from build123d import *

# Parameters (mm, degrees)
F0_R     = 5.5
F0_R_2   = 42
F1_DEPTH = 12


with BuildPart() as f1:
    # F0 (on Front) → F1 (new body)
    with BuildSketch(Plane.XZ):
        with BuildLine():
            ThreePointArc((-52.973189, -28.214553), (-49.277102, -27.650029), (-46.222895, -29.806777))
            ThreePointArc((-46.222895, -29.806777), (-32.248964, -44.553388), (-13.874959, -53.2211))
            ThreePointArc((-13.874959, -53.2211), (-10.872022, -55.44868), (-10.253636, -59.136137))
            ThreePointArc((-10.253636, -59.136137), (0, -71.897322), (10.253636, -59.136137))
            ThreePointArc((10.253636, -59.136137), (10.872022, -55.44868), (13.874959, -53.2211))
            ThreePointArc((13.874959, -53.2211), (32.248964, -44.553388), (46.222895, -29.806777))
            ThreePointArc((46.222895, -29.806777), (49.277102, -27.650029), (52.973189, -28.214553))
            ThreePointArc((52.973189, -28.214553), (68.298918, -22.460693), (59.379651, -8.733655))
            ThreePointArc((59.379651, -8.733655), (56.069932, -6.994258), (54.891958, -3.44572))
            ThreePointArc((54.891958, -3.44572), (47.477641, 27.764611), (23.912186, 49.529864))
            ThreePointArc((23.912186, 49.529864), (21.397105, 52.29647), (21.504018, 56.033891))
            ThreePointArc((21.504018, 56.033891), (13.913807, 70.538152), (1.384423, 60.002526))
            ThreePointArc((1.384423, 60.002526), (0.064118, 56.504449), (-3.313139, 54.900119))
            ThreePointArc((-3.313139, 54.900119), (-41.207009, 36.42777), (-54.891958, -3.44572))
            ThreePointArc((-54.891958, -3.44572), (-56.069932, -6.994258), (-59.379651, -8.733655))
            ThreePointArc((-59.379651, -8.733655), (-68.298918, -22.460693), (-52.973189, -28.214553))
        make_face()
        with Locations((-58.324435, -19.180497)):
            Circle(F0_R, mode=Mode.SUBTRACT)
        with Locations((0, -61.397322)):
            Circle(F0_R, mode=Mode.SUBTRACT)
        with Locations((58.324435, -19.180497)):
            Circle(F0_R, mode=Mode.SUBTRACT)
        Circle(F0_R_2, mode=Mode.SUBTRACT)
        with Locations((11.881813, 60.236647)):
            Circle(F0_R, mode=Mode.SUBTRACT)
    extrude(amount=F1_DEPTH)


solid = f1.part
Geometry check sheet. Reference: the model listing, model coordinates, mm. Round coordinates to 2 decimals unless told otherwise and drop trailing zeros. Write each loop counter-clockwise with the first axis right and the second up, starting at its lowest first coordinate (ties: lowest second). Pieces come first, ordered by that corner, then holes.
Item 1: Material ranges on line 1 along Z through (x, y) = (13.5, -7); line 2 along X through (y, z) = (-3.25, -58.5); line 3 along Z through (x, y) = (15, -1.25), recorded low to high.
Determined:
line 1: z = -53.33 to -39.77, 39.77 to 54.98, 65.49 to 70.61
line 2: x = -10.16 to -4.67, 4.67 to 10.16
line 3: z = -52.92 to -39.23, 39.23 to 55.71, 64.77 to 70.26
Item 2: Section check B-B (x = -0.5). Record the boundary of the cut face in (y, z).
Determined:
outline: (-12, -71.89) - (0, -71.89) - (0, -66.87) - (-12, -66.87) - close; (-12, -55.92) - (0, -55.92) - (0, -42) - (-12, -42) - close; (-12, 42) - (0, 42) - (0, 55.98) - (-12, 55.98) - close
Item 3: Go/stop test with flat-tipped pins: pin 1 Ø1.5 at (x, y) = (8.5, -8.5) entering from +Z; pin 2 Ø6 at (y, z) = (-5.5, 22.5) entering from +X; pin 3 Ø1 at (x, y) = (-38.5, -1.5) entering from -Z. Record where each tip stops, or that it passes through.
Determined:
pin 1: stops at z = 70.4
pin 2: stops at x = 51.43
pin 3: stops at z = -39.76
Item 4: Section check D-D (y = -8.25). Record the boundary of the cut face in (x, z), plus the area to 3 significant figures.
Determined:
outline: (-59.38, -8.73) arc R10.5 ccw (long way) to (-52.97, -28.21) arc R5 cw to (-46.22, -29.81) arc R55 ccw to (-13.87, -53.22) arc R5 cw to (-10.25, -59.14) arc R10.5 ccw (long way) to (10.25, -59.14) arc R5 cw to (13.87, -53.22) arc R55 ccw to (46.22, -29.81) arc R5 cw to (52.97, -28.21) arc R10.5 ccw (long way) to (59.38, -8.73) arc R5 cw to (54.89, -3.45) arc R55 ccw to (23.91, 49.53) arc R5 cw to (21.5, 56.03) arc R10.5 ccw (long way) to (1.38, 60) arc R5 cw to (-3.31, 54.9) arc R55 ccw to (-54.89, -3.45) arc R5 cw to start; hole circle Ø11 at (-58.32, -19.18); hole circle Ø84 at (0, 0); hole circle Ø11 at (0, -61.4); hole circle Ø11 at (11.88, 60.24); hole circle Ø11 at (58.32, -19.18)
area: 4,850 mm2
Item 5: Mould release check, pull along X, two halves, no side actions. Record for faces 1 (the face through (10.844, -5.916, -55.495)), 2 (the face through (-1.192, -5.916, -66.767)), 3 (the face through (5, 0, 42)): +X half, -X half, draft (parallel to the pull), parting line (faces both ways), or undercut.
Determined:
face 1: +X half
face 2: undercut
face 3: draft
Item 6: Section check A-A (z = 0). Record the boundary of the cut face in (x, y), plus the area to 3 significant figures.
Determined:
outline: (-55, -12) - (-42, -12) - (-42, 0) - (-55, 0) - close; (42, -12) - (55, -12) - (55, 0) - (42, 0) - close
area: 312 mm2
Item 7: Section check C-C (x = -57.5). Record the boundary of the cut face in (y, z), plus the area to 3 significant figures.
Determined:
outline: (-12, -29.65) - (0, -29.65) - (0, -24.62) - (-12, -24.62) - close; (-12, -13.74) - (0, -13.74) - (0, -8.16) - (-12, -8.16) - close
area: 127 mm2
